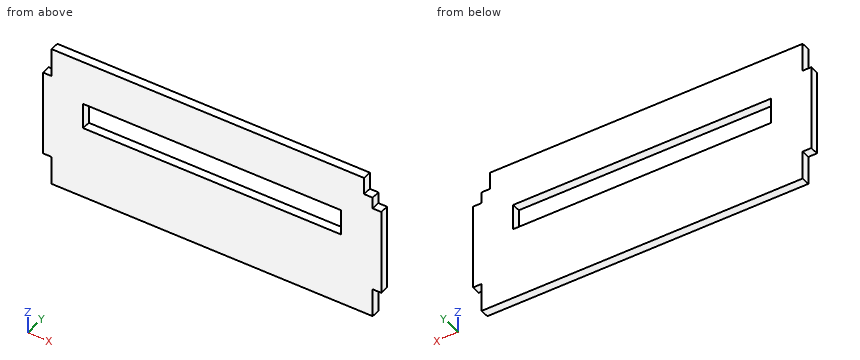
```python
from build123d import *

# Parameters (mm, degrees)
LED_1_OUTLINE_R     = 2.25
LED_1_DEPTH         = 3
SKETCH_1_W          = 90
SKETCH_1_H          = 9
CUT_EXTRUDE_1_DEPTH = 3


# Read off the part's stored shape, not the designer's step: 基体零件-LED板-1
with BuildPart() as part:
    # 基体零件-LED板-1 outline → 基体零件-LED板-1 (new body)
    with BuildSketch(Plane(origin=(0, 0, 0), x_dir=(1, 0, 0), z_dir=(0, 1, 0))):
        Polygon((-3, -140), (0, -140), (0, -110), (-3, -110), (-3, -100), (-115, -100), (-115, -110), (-118, -110), (-118, -140), (-115, -140), (-115, -150), (-6.001970153, -150), (-6.001970153, -144), (-3, -144), align=None)
        with Locations((-90.5, -130)):
            Circle(LED_1_OUTLINE_R, mode=Mode.SUBTRACT)
        with Locations((-81.5, -130)):
            Circle(LED_1_OUTLINE_R, mode=Mode.SUBTRACT)
        with Locations((-72.5, -130)):
            Circle(LED_1_OUTLINE_R, mode=Mode.SUBTRACT)
        with Locations((-63.5, -130)):
            Circle(LED_1_OUTLINE_R, mode=Mode.SUBTRACT)
        with Locations((-54.5, -130)):
            Circle(LED_1_OUTLINE_R, mode=Mode.SUBTRACT)
        with Locations((-45.5, -130)):
            Circle(LED_1_OUTLINE_R, mode=Mode.SUBTRACT)
        with Locations((-36.5, -130)):
            Circle(LED_1_OUTLINE_R, mode=Mode.SUBTRACT)
        with Locations((-27.5, -130)):
            Circle(LED_1_OUTLINE_R, mode=Mode.SUBTRACT)
    extrude(amount=LED_1_DEPTH)

    # 草图1 → 切除-拉伸1 (cut)
    with BuildSketch(Plane(origin=(0, 3, 0), x_dir=(1, 0, 0), z_dir=(0, 1, 0))):
        with Locations((-59, -130)):
            Rectangle(SKETCH_1_W, SKETCH_1_H)
    extrude(amount=-CUT_EXTRUDE_1_DEPTH, mode=Mode.SUBTRACT)


solid = part.part
```
Geometry: final body of the model. Coordinates: model frame, mm. Coordinates: 2 decimals unless noted, no trailing zeros. Loops run counter-clockwise (first coordinate to the right, second up) from the corner with the lowest first, then second, coordinate; pieces in that order, holes last. Notation, with made-up numbers: M -14.75,67.5 L 15.25,67.5 A12 ccw 15.25,86.5 Z; hole C 51.5,87 d4. An arc over 180 degrees is marked long. Put each result on its own line as item: value.
(1) Cut plane A-A on y = 1.6. Return the cut outline in (x, z), then the cut area to 3 significant figures.
Answer sheet:
outline: M -118,110 L -115,110 L -115,100 L -3,100 L -3,110 L 0,110 L 0,140 L -3,140 L -3,144 L -6,144 L -6,150 L -115,150 L -115,140 L -118,140 Z; hole M -104,125.5 L -14,125.5 L -14,134.5 L -104,134.5 Z
area: 4,950 mm^2
(2) Material intervals for probe 1 along Z at (x, y) = (-22.5, 0.8); probe 2 along X at (y, z) = (1.45, 126); probe 3 along X at (y, z) = (2.8, 145), sorted ascending.
Answer sheet:
probe 1: z = 100 to 125.5, 134.5 to 150
probe 2: x = -118 to -104, -14 to 0
probe 3: x = -115 to -6
(3) Cut plane B-B on z = 127.5. Return the cut outline in (x, y), then the cut area to 3 significant figures.
Answer sheet:
outline: M -118,0 L -104,0 L -104,3 L -118,3 Z; M -14,0 L 0,0 L 0,3 L -14,3 Z
area: 84.0 mm^2
(4) Cut plane C-C on x = -98. Return the cut outline in (y, z).
Answer sheet:
outline: M 0,100 L 3,100 L 3,125.5 L 0,125.5 Z; M 0,134.5 L 3,134.5 L 3,150 L 0,150 Z
(5) First-contact query: pin 1 (1.5 mm diameter, centred on y = 1, z = 105, fed in from -X); pin 2 (1.5 mm diameter, centred on x = -4, y = 2, fed in from +Z); pin 3 (1.5 mm diameter, centred on x = -117, y = 1, fed in from +Z). Flat tips, straight axial feed; report the tip coordinate or a pass-through.
Answer sheet:
pin 1: stops at x = -115
pin 2: stops at z = 144
pin 3: stops at z = 140
(6) Cut plane D-D on z = 147.5. Return the cut outline in (x, y).
Answer sheet:
outline: M -115,0 L -6,0 L -6,3 L -115,3 Z
